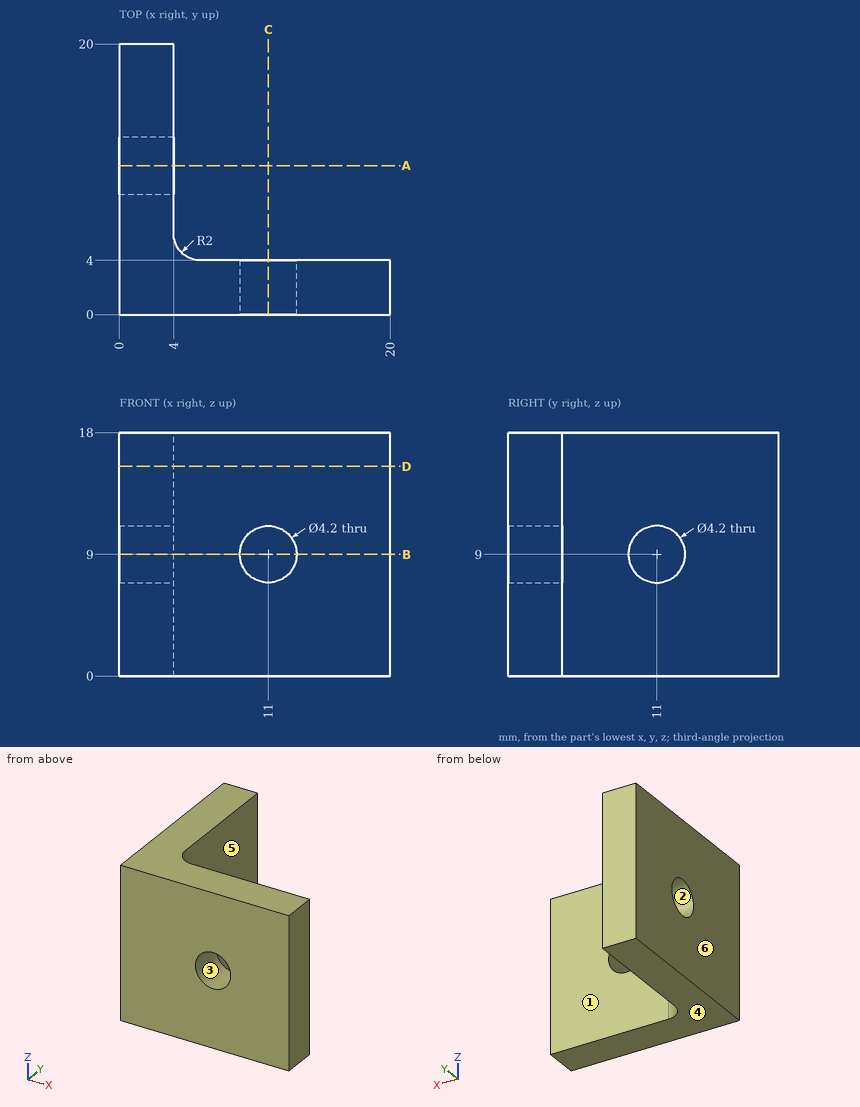
Drawing for the job (mm, zero at the part's lowest x, y, z). A direction names the side the tool comes from. Coordinates: 2 decimals unless noted, no trailing zeros. Loops run counter-clockwise (first coordinate to the right, second up) from the corner with the lowest first, then second, coordinate; pieces in that order, holes last. Notation, with made-up numbers: (77.5, 48) - (120.5, 48) arc R18 ccw to (120.5, 54) - close; hole circle Ø5 at (57.25, 34.25). An arc over 180 degrees is marked (long way). Use CSV: the item, a comma, the result in double quotes. Start each with the question number.
Q1. Cut at A-A, the plane y = 11. List the corners of the cut face in (x, z), then the cut area to 3 significant figures.
Q2. Probe probe 1 along Z at (x, y) = (11, 1.7); probe 2 along Y at (x, z) = (16.5, 2.75). List the from-to ranges inside material, lowest first. Write a range as from..to.
Q3. Drop flat-ended pins along their axis: P1, Ø7, axis at y = 13, z = 8, coming from the +X side; P2, Ø2.5, axis at y = 11, z = 9, coming from the -X side; P3, Ø10, axis at x = 18, z = 10.5, coming from the +Y side. Give the stop position or say it passes through.
Q4. 3-axis set-ups, long thin cutter, end or side, ignore diameter. For the marked faces 5 and 6: which of +Z, -Z, +X, -X, +Y, -Y reach the whole face in a straight line?
Q5. Cut at B-B, the plane z = 9. List the corners of the cut face in (x, y), then the cut area to 3 significant figures.
Q6. Cut at D-D, the plane z = 15.5. List the corners of the cut face in (x, y), then the cut area to 3 significant figures.
Q7. Two-plate mould, pull along Z, no slides. Class the marked faces 1, 2, 3 and 4: +Z half, -Z half, draft (parallel to the pull), parting line (faces both ways), or undercut.
Here are the results:
1,outline,"(0, 0) - (4, 0) - (4, 6.9) - (0, 6.9) - close; (0, 11.1) - (4, 11.1) - (4, 18) - (0, 18) - close"
1,area,"55.2 mm2"
2,probe 1,"0..6.9, 11.1..18"
2,probe 2,"0..4"
3,P1,"x = 4"
3,P2,"through"
3,P3,"y = 4"
4,face 5,"+Z, -Z, +X, +Y"
4,face 6,"+Z, -Z, -X, +Y, -Y"
5,outline,"(0, 0) - (8.9, 0) - (8.9, 4) - (6, 4) arc R2 cw to (4, 6) - (4, 8.9) - (0, 8.9) - close; (0, 13.1) - (4, 13.1) - (4, 20) - (0, 20) - close; (13.1, 0) - (20, 0) - (20, 4) - (13.1, 4) - close"
5,area,"111 mm2"
6,outline,"(0, 0) - (20, 0) - (20, 4) - (6, 4) arc R2 cw to (4, 6) - (4, 20) - (0, 20) - close"
6,area,"145 mm2"
7,face 1,"draft"
7,face 2,"undercut"
7,face 3,"undercut"
7,face 4,"-Z half"
